```python
from build123d import *

# Parameters (mm, degrees)
SKETCH1_W           = 45
SKETCH1_H           = 25
BOSS_EXTRUDE1_DEPTH = 5
SKETCH2_R           = 1.5
CUT_EXTRUDE1_DEPTH  = 27.220221204
CUT_EXTRUDE2_DEPTH  = 27.220221204
CHAMFER2_SIZE       = 2
BOSS_EXTRUDE2_DEPTH = 5
FILLET1_R           = 1


with BuildPart() as part:
    # Sketch1 → Boss-Extrude1 (new body)
    with BuildSketch(Plane(origin=(0, 0, 0), x_dir=(0, 0, -1), z_dir=(1, 0, 0))):
        Rectangle(SKETCH1_W, SKETCH1_H)
    extrude(amount=BOSS_EXTRUDE1_DEPTH)

    # Sketch2 → Cut-Extrude1 (cut, through all)
    with BuildSketch(Plane(origin=(5, 0, 0), x_dir=(0, 0, -1), z_dir=(1, 0, 0))):
        with Locations((-18.5, -9.5)):
            Circle(SKETCH2_R)
        with Locations((18.5, -9.5)):
            Circle(SKETCH2_R)
    extrude(amount=-CUT_EXTRUDE1_DEPTH, mode=Mode.SUBTRACT)

    # Sketch3 → Cut-Extrude2 (cut, through all)
    with BuildSketch(Plane(origin=(5, 0, 0), x_dir=(0, 0, -1), z_dir=(1, 0, 0))):
        Polygon((-12.5, 9.80361421), (-12.5, -5.599476508), (2.5, -5.599476508), align=None)
        Polygon((-2.5, 9.80361421), (12.5, 9.80361421), (12.5, -5.599476508), align=None)
    extrude(amount=-CUT_EXTRUDE2_DEPTH, mode=Mode.SUBTRACT)

    # Chamfer2
    chamfer2_edges = [part.edges().sort_by_distance(p)[0] for p in [
        (0, 0, 22.5),
        (0, 0, -22.5),
    ]]
    chamfer(chamfer2_edges, length=CHAMFER2_SIZE)

    # Sketch4 → Boss-Extrude2 (add)
    with BuildSketch(Plane(origin=(0, 0, -22.5), x_dir=(-1, 0, 0), z_dir=(0, 0, -1))):
        Polygon((-5, -5), (-21.490292585, -5), (-5, 11.490292585), align=None)
    extrude(amount=-BOSS_EXTRUDE2_DEPTH)

    # Fillet1
    fillet1_edges = [part.edges().sort_by_distance(p)[0] for p in [
        (5, 11.490292585, -20),
        (21.490292585, -5, -20),
    ]]
    fillet(fillet1_edges, radius=FILLET1_R)


solid = part.part
```
For this review, take the finished solid that the model builds, in its own axes (mm). A direction names the side the tool comes from. Give positions to 0.01 mm unless a question says otherwise; leave off trailing zeros. Write each loop counter-clockwise with the first axis right and the second up, starting at its lowest first coordinate (ties: lowest second). Pieces come first, ordered by that corner, then holes. Notation, with made-up numbers: M 27.5,25.5 L 66.5,25.5 A12 cw 66.5,48.5 Z; hole C 66,71 d6. An arc over 180 degrees is marked long. Answer as CSV lines item,"result".
1. For pin 1 (7.5 mm diameter, centred on y = 3, z = 2, fed in from +X); pin 2 (1.5 mm diameter, centred on x = 13, z = -19.5, fed in from -Y), all flat-tipped, find the tip position at first contact; note any pin that passes through.
Findings:
pin 1,"stops at x = 5"
pin 2,"stops at y = -5"
2. Consider section A-A, the plane z = -18.5. Write out the cut boundary in (x, y).
Findings:
outline,"M 0,-12.5 L 5,-12.5 L 5,-11 L 0,-11 Z; M 0,-8 L 5,-8 L 5,-5 L 19.08,-5 A1 ccw 19.78,-3.29 L 5.29,11.2 A1 cw 5,11.9 L 5,12.5 L 0,12.5 Z"
3. Consider section B-B, the plane y = 2.5. Write out the cut boundary in (x, z).
Findings:
outline,"M 0,-20.5 L 2,-22.5 L 13.99,-22.5 L 13.99,-17.5 L 5,-17.5 L 5,-12.5 L 0,-12.5 Z; M 0,-4.61 L 5,-4.61 L 5,5.39 L 0,5.39 Z; M 0,12.5 L 5,12.5 L 5,22.5 L 2,22.5 L 0,20.5 Z"
4. Consider section D-D, the plane z = 18.5. Write out the cut boundary in (x, y), then the cut area to 3 significant figures.
Findings:
outline,"M 0,-12.5 L 5,-12.5 L 5,-11 L 0,-11 Z; M 0,-8 L 5,-8 L 5,12.5 L 0,12.5 Z"
area,"110 mm2"
5. Consider section C-C, the plane x = 3.5. Write out the cut boundary in (y, z).
Findings:
outline,"M -12.5,-22.5 L 12.5,-22.5 L 12.5,22.5 L -12.5,22.5 Z; hole C -9.5,-18.5 d3; hole C -9.5,18.5 d3; hole M -5.6,-12.5 L 9.8,-12.5 L 9.8,2.5 Z; hole M -5.6,-2.5 L 9.8,12.5 L -5.6,12.5 Z"
6. For faces 1 (the cylindrical face through (20.006, -4.367, -19.965)), 2 (the flat face through (3, 2, 12.5)), 3 (the flat face through (11, 0, -17.5)), list the 3-axis set-ups (+Z, -Z, +X, -X, +Y, -Y) from which the entire face can be reached by the end or side of a thin tool; tool diameter is ignored.
Findings:
face 1,"+Z, -Z, +X"
face 2,"+X, -X"
face 3,"+Z, +X, +Y, -Y"
7. Draft analysis for pull direction Y (two halves, no side actions). For faces 4 (the flat face through (3, -5.599, 5)), 5 (the flat face through (12, -5, -20)), 6 (the flat face through (5, 0, 0)), state which applies: +Y half, -Y half, draft (parallel to the pull), parting line (faces both ways), or undercut.
Findings:
face 4,"undercut"
face 5,"-Y half"
face 6,"draft"
8. Wall thickness on line 1 (Y direction, x = 2.5, z = -18.5); line 2 (Z direction, x = 13, y = -1.25); line 3 (X direction, y = -8.5, z = -0.5): over which ranges is each line inside the solid? List them lowest first.
Findings:
line 1,"y = -12.5 to -11, -8 to 12.5"
line 2,"z = -22.5 to -17.5"
line 3,"x = 0 to 5"
